from build123d import *

# Parameters (mm, degrees)
BOSS_EXTRU_1_DEPTH      = 39.2
ESQUISSE2_W             = 20.710678119
ESQUISSE2_H             = 1.4
ESQUISSE2_W_2           = 1.4
ESQUISSE2_H_2           = 20.710678119
ENL_V_MAT_EXTRU_1_DEPTH = 15
ESQUISSE3_R             = 1.7
ENL_V_MAT_EXTRU_2_DEPTH = 108.408751971
ENL_V_START             = -5
ESQUISSE4_R             = 3.5
ENL_V_MAT_EXTRU_3_DEPTH = 103.408751971
ESQUISSE5_R             = 1.25
ENL_V_MAT_EXTRU_4_DEPTH = 103.408751971
ESQUISSE6_R             = 12.5
ENL_V_MAT_EXTRU_5_DEPTH = 108.408751971
ESQUISSE7_OUTSIDE_W     = 184.184
ESQUISSE7_OUTSIDE_H     = 184.184
ESQUISSE7_OUTSIDE_R     = 24.5
ESQUISSE7_OUTSIDE_R_2   = 4.75
ENL_V_MAT_EXTRU_6_DEPTH = 108.408751971


with BuildPart() as part:
    # Esquisse1 → Boss.-Extru.1 (new body)
    with BuildSketch(Plane(origin=(0, 0, 0), x_dir=(1, 0, 0), z_dir=(0, 1, 0))):
        Polygon((0, 70.710678119), (70.710678119, 0), (0, -70.710678119), (-70.710678119, 0), align=None)
    extrude(amount=BOSS_EXTRU_1_DEPTH)

    # Esquisse2 → Enlèv. mat.-Extru.1 (cut)
    with BuildSketch(Plane(origin=(0, 39.2, 0), x_dir=(1, 0, 0), z_dir=(0, 1, 0))):
        with Locations((55.35533906, 0)):
            Rectangle(ESQUISSE2_W, ESQUISSE2_H)
        with Locations((0, 55.35533906)):
            Rectangle(ESQUISSE2_W_2, ESQUISSE2_H_2)
        with Locations((-55.35533906, 0)):
            Rectangle(ESQUISSE2_W, ESQUISSE2_H)
    extrude(amount=-ENL_V_MAT_EXTRU_1_DEPTH, mode=Mode.SUBTRACT)

    # Esquisse3 → Enlèv. mat.-Extru.2 (cut, through all)
    with BuildSketch(Plane(origin=(0, 39.2, 0), x_dir=(1, 0, 0), z_dir=(0, 1, 0))):
        with Locations(Location((20.859650045, 20.859650045, 0), (0, 0, 270))):
            Circle(ESQUISSE3_R)
        with Locations(Location((20.859650045, -20.859650045, 0), (0, 0, 270))):
            Circle(ESQUISSE3_R)
        with Locations(Location((-20.859650045, 20.859650045, 0), (0, 0, 270))):
            Circle(ESQUISSE3_R)
        with Locations(Location((-20.859650045, -20.859650045, 0), (0, 0, 270))):
            Circle(ESQUISSE3_R)
    extrude(amount=-ENL_V_MAT_EXTRU_2_DEPTH, mode=Mode.SUBTRACT)

    # Esquisse4 → Enlèv. mat.-Extru.3 (cut, through all)
    with BuildSketch(Plane(origin=(0, 39.2, 0), x_dir=(1, 0, 0), z_dir=(0, 1, 0)).offset(ENL_V_START)):
        with Locations(Location((20.859650045, 20.859650045, 0), (0, 0, 270))):
            Circle(ESQUISSE4_R)
        with Locations(Location((20.859650045, -20.859650045, 0), (0, 0, 270))):
            Circle(ESQUISSE4_R)
        with Locations(Location((-20.859650045, 20.859650045, 0), (0, 0, 270))):
            Circle(ESQUISSE4_R)
        with Locations(Location((-20.859650045, -20.859650045, 0), (0, 0, 270))):
            Circle(ESQUISSE4_R)
    extrude(amount=-ENL_V_MAT_EXTRU_3_DEPTH, mode=Mode.SUBTRACT)

    # Esquisse5 → Enlèv. mat.-Extru.4 (cut, through all)
    with BuildSketch(Plane(origin=(0, 39.2, 0), x_dir=(1, 0, 0), z_dir=(0, 1, 0)).offset(ENL_V_START)):
        with Locations(Location((29.5, 0, 0), (0, 0, 270))):
            Circle(ESQUISSE5_R)
        with Locations(Location((-29.5, 0, 0), (0, 0, 270))):
            Circle(ESQUISSE5_R)
        with Locations(Location((0, -29.5, 0), (0, 0, 270))):
            Circle(ESQUISSE5_R)
        with Locations(Location((0, 29.5, 0), (0, 0, 270))):
            Circle(ESQUISSE5_R)
    extrude(amount=-ENL_V_MAT_EXTRU_4_DEPTH, mode=Mode.SUBTRACT)

    # Esquisse6 → Enlèv. mat.-Extru.5 (cut, through all)
    with BuildSketch(Plane(origin=(0, 39.2, 0), x_dir=(1, 0, 0), z_dir=(0, 1, 0))):
        with Locations(Location((0, -48.790367902, 0), (0, 0, 270))):
            Circle(ESQUISSE6_R)
    extrude(amount=-ENL_V_MAT_EXTRU_5_DEPTH, mode=Mode.SUBTRACT)

    # Esquisse7 outside → Enlèv. mat.-Extru.6 (cut, through all)
    # profile 1 of 10: a face of its own
    with BuildSketch(Plane(origin=(0, 39.2, 0), x_dir=(1, 0, 0), z_dir=(0, 1, 0))):
        Rectangle(ESQUISSE7_OUTSIDE_W, ESQUISSE7_OUTSIDE_H)
        with BuildLine():
            Line((5, 41.821047333), (5, 63.639610307))
            ThreePointArc((5, 63.639610307), (0, 68.639610307), (-5, 63.639610307))
            Line((-5, 63.639610307), (-5, 41.821047333))
            ThreePointArc((-5, 41.821047333), (-6.074827807, 38.723786728), (-8.837209302, 36.958134852))
            ThreePointArc((-8.837209302, 36.958134852), (-26.870057685, 26.870057685), (-36.958134852, 8.837209302))
            ThreePointArc((-36.958134852, 8.837209302), (-38.723786728, 6.074827807), (-41.821047333, 5))
            Line((-41.821047333, 5), (-63.639610307, 5))
            ThreePointArc((-63.639610307, 5), (-68.639610307, 0), (-63.639610307, -5))
            Line((-63.639610307, -5), (-41.821047333, -5))
            ThreePointArc((-41.821047333, -5), (-38.723786728, -6.074827807), (-36.958134852, -8.837209302))
            ThreePointArc((-36.958134852, -8.837209302), (-30.152523014, -23.126291443), (-18.11627907, -33.403599097))
            ThreePointArc((-18.11627907, -33.403599097), (-16.20357098, -35.241330732), (-15.5, -37.798809505))
            Line((-15.5, -37.798809505), (-15.5, -48.790367902))
            ThreePointArc((-15.5, -48.790367902), (0, -64.290367902), (15.5, -48.790367902))
            Line((15.5, -48.790367902), (15.5, -37.798809505))
            ThreePointArc((15.5, -37.798809505), (16.20357098, -35.241330732), (18.11627907, -33.403599097))
            ThreePointArc((18.11627907, -33.403599097), (30.152523014, -23.126291443), (36.958134852, -8.837209302))
            ThreePointArc((36.958134852, -8.837209302), (38.723786728, -6.074827807), (41.821047333, -5))
            Line((41.821047333, -5), (63.639610307, -5))
            ThreePointArc((63.639610307, -5), (68.639610307, 0), (63.639610307, 5))
            Line((63.639610307, 5), (41.821047333, 5))
            ThreePointArc((41.821047333, 5), (38.723786728, 6.074827807), (36.958134852, 8.837209302))
            ThreePointArc((36.958134852, 8.837209302), (26.870057685, 26.870057685), (8.837209302, 36.958134852))
            ThreePointArc((8.837209302, 36.958134852), (6.074827807, 38.723786728), (5, 41.821047333))
        make_face(mode=Mode.SUBTRACT)
    # profile 2 of 10: a face of its own
    with BuildSketch(Plane(origin=(0, 39.2, 0), x_dir=(1, 0, 0), z_dir=(0, 1, 0))):
        with Locations(Location((0, 0, 0), (0, 0, 270))):
            Circle(ESQUISSE7_OUTSIDE_R)
    # profile 3 of 10: a face of its own
    with BuildSketch(Plane(origin=(0, 39.2, 0), x_dir=(1, 0, 0), z_dir=(0, 1, 0))):
        with Locations(Location((11.958857261, 28.871235391, 0), (0, 0, 270))):
            Circle(ESQUISSE7_OUTSIDE_R_2)
    # profile 4 of 10: a face of its own
    with BuildSketch(Plane(origin=(0, 39.2, 0), x_dir=(1, 0, 0), z_dir=(0, 1, 0))):
        with Locations(Location((28.871235391, 11.958857261, 0), (0, 0, 270))):
            Circle(ESQUISSE7_OUTSIDE_R_2)
    # profile 5 of 10: a face of its own
    with BuildSketch(Plane(origin=(0, 39.2, 0), x_dir=(1, 0, 0), z_dir=(0, 1, 0))):
        with Locations(Location((28.871235391, -11.958857261, 0), (0, 0, 270))):
            Circle(ESQUISSE7_OUTSIDE_R_2)
    # profile 6 of 10: a face of its own
    with BuildSketch(Plane(origin=(0, 39.2, 0), x_dir=(1, 0, 0), z_dir=(0, 1, 0))):
        with Locations(Location((11.958857261, -28.871235391, 0), (0, 0, 270))):
            Circle(ESQUISSE7_OUTSIDE_R_2)
    # profile 7 of 10: a face of its own
    with BuildSketch(Plane(origin=(0, 39.2, 0), x_dir=(1, 0, 0), z_dir=(0, 1, 0))):
        with Locations(Location((-11.958857261, -28.871235391, 0), (0, 0, 270))):
            Circle(ESQUISSE7_OUTSIDE_R_2)
    # profile 8 of 10: a face of its own
    with BuildSketch(Plane(origin=(0, 39.2, 0), x_dir=(1, 0, 0), z_dir=(0, 1, 0))):
        with Locations(Location((-28.871235391, -11.958857261, 0), (0, 0, 270))):
            Circle(ESQUISSE7_OUTSIDE_R_2)
    # profile 9 of 10: a face of its own
    with BuildSketch(Plane(origin=(0, 39.2, 0), x_dir=(1, 0, 0), z_dir=(0, 1, 0))):
        with Locations(Location((-28.871235391, 11.958857261, 0), (0, 0, 270))):
            Circle(ESQUISSE7_OUTSIDE_R_2)
    # profile 10 of 10: a face of its own
    with BuildSketch(Plane(origin=(0, 39.2, 0), x_dir=(1, 0, 0), z_dir=(0, 1, 0))):
        with Locations(Location((-11.958857261, 28.871235391, 0), (0, 0, 270))):
            Circle(ESQUISSE7_OUTSIDE_R_2)
    extrude(amount=-ENL_V_MAT_EXTRU_6_DEPTH, mode=Mode.SUBTRACT)


solid = part.part
The listing builds one solid part. Answer for the finished solid, in the listing's coordinates (mm). A direction names the side the tool comes from. Give positions to 0.01 mm unless a question says otherwise; leave off trailing zeros. Loops run counter-clockwise (first coordinate to the right, second up) from the corner with the lowest first, then second, coordinate; pieces in that order, holes last. Notation, with made-up numbers: (-34, 21.25) - (11, 21.25) arc R22 cw to (11, 40.25) - close; hole circle Ø5 at (-2.5, 56). An arc over 180 degrees is marked (long way). Answer as a JSON object with one key per item and string values.
1. A cutting plane is placed at B-B (y = 16). Give the number of separate pieces and of enclosed holes in the cut face, then the cut area to 3 significant figures.
Determined:
{"separate pieces": "1", "enclosed holes": "18", "area": "3,080 mm²"}
2. Find the intervals of material crossed by L1, parallel to X at y = 10.5, z = 0; L2, parallel to X at y = 8.5, z = -0.5; L3, parallel to Z at x = -29, y = 15, in increasing order. Write a range as [from, to].
Determined:
{"L1": "[-68.64, -30.75], [-28.25, -24.5], [24.5, 28.25], [30.75, 68.64]", "L2": "[-68.61, -30.65], [-28.35, -24.49], [24.49, 28.35], [30.65, 68.61]", "L3": "[-24.56, -16.71], [-7.21, -1.15], [1.15, 7.21], [16.71, 24.56]"}
3. For a pull along X with two mould halves and no side action, classify faces 4 (the cylindrical face through (-20.706, 17.339, 17.363)), 5 (the cylindrical face through (68.64, 19.87, 0.11)), 6 (the cylindrical face through (-6.046, 19.874, -38.761)) as pulls with the +X half, pulls with the -X half, needs draft (parallel to the pull), parting line crosses it, or undercut.
Determined:
{"face 4": "undercut", "face 5": "pulls with the +X half", "face 6": "pulls with the -X half"}
4. For faces 1 (the flat face through (-15.5, 20, 43)), 2 (the flat face through (19, 34.2, 20)), 3 (the cylindrical face through (19.83, 36.74, -22.21)), determine the directions among +Z, -Z, +X, -X, +Y, -Y from which every point of the face is accessible in a straight line to the end or side of a thin tool.
Determined:
{"face 1": "+Z, -X, +Y, -Y", "face 2": "-Y", "face 3": "+Y, -Y"}
5. A cutting plane is placed at A-A (z = 14). Write down the section's boundary in (x, y).
Determined:
{"outline": "(-35.33, 0) - (-33.16, 0) - (-33.16, 39.2) - (-35.33, 39.2) - close; (-24.58, 0) - (-20.11, 0) - (-20.11, 39.2) - (-24.58, 39.2) - close; (20.11, 0) - (24.58, 0) - (24.58, 39.2) - (20.11, 39.2) - close; (33.16, 0) - (35.33, 0) - (35.33, 39.2) - (33.16, 39.2) - close"}
6. Flat-ended cylindrical pins translate along their axes: pin 1 Ø12 at (x, y) = (52, 29.5) entering from +Z; pin 2 Ø2 at (x, z) = (0, 29.5) entering from -Y; pin 3 Ø1.5 at (x, z) = (-29, 1.5) entering from -Y; pin 4 Ø1 at (y, z) = (28, -27) entering from +X. Find the tip coordinate at first contact, or state that the pin passes through.
Determined:
{"pin 1": "z = 5", "pin 2": "y = 34.2", "pin 3": "y = 0", "pin 4": "x = 27.24"}
